Here's how the part is built. I have some questions about the finished solid (model axes, mm). A direction names the side the tool comes from. Round coordinates to 2 decimals unless told otherwise and drop trailing zeros. Write each loop counter-clockwise with the first axis right and the second up, starting at its lowest first coordinate (ties: lowest second). Pieces come first, ordered by that corner, then holes. Notation, with made-up numbers: (8.5, 22.5) - (51.5, 22.5) arc R27 ccw to (51.5, 39.5) - close; hole circle Ø10 at (6, 65.25). An arc over 180 degrees is marked (long way). One line per item, written item: value. Start each with the question number.
Item 1: If I drill on line 1 (X direction, y = 0, z = -0.2); line 2 (X direction, y = 0, z = -2.8); line 3 (Z direction, x = 2.75, y = 2.25), over which ranges is the centre line in solid material (lowest first)?
Item 2: Imagine slicing it at D-D, the plane x = -2.75. Please give me the cut outline in (y, z), then the cut area to 3 significant figures.
Item 3: For faces 3 (the face through (-2.75, 1.43, -4.05)), 4 (the face through (2.44, -0.54, -2.07)), which set-ups out of +Z, -Z, +X, -X, +Y, -Y let a thin tool reach every point of the face, with its end or its side?
Item 4: Imagine slicing it at C-C, the plane z = -1.3. Please give me the cut outline in (x, y).
Item 5: Imagine slicing it at A-A, the plane x = 0. Please give me the cut outline in (y, z).
Item 6: Thinking about a two-plate mould opening in Y: for faces 1 (the face through (-4.88, -1.08, -2.13)), 2 (the face through (2.8, -3.65, -4.05)), which applies, released by +Y, released by -Y, zero draft, split by the parting line, or undercut?
Autodesk Inventor part; units mm, degrees
ref_plane "YZ Plane" through (0, 0, 0) normal (1, 0, 0) x (0, 1, 0)
ref_plane "XZ Plane" through (0, 0, 0) normal (0, 1, 0) x (-1, 0, 0)
ref_plane "XY Plane" through (0, 0, 0) normal (0, 0, 1) x (1, 0, 0)
sketch "Sketch1" plane through (0, 0, 0) normal (1, 0, 0) x (0, 1, 0)
  line L0 (4, 0) -> (2.5, 0)
  line L1 (2.5, 0) -> (3.1, 0)
  line L2 (3.1, 0) -> (3.1, -0.3)
  line L3 (3.1, -0.3) -> (4.6, -0.3)
  line L4 (4.6, -0.3) -> (4.6, 0)
  line L5 (4.6, 0) -> (5, 0)
  line L6 (5, 0) -> (5, -4.2)
  line L7 (5, -4.2) -> (4.6, -4.2)
  line L8 (4.6, -4.2) -> (4.6, -3.9)
  line L9 (4.6, -3.9) -> (3.1, -3.9)
  line L10 (3.1, -3.9) -> (3.1, -4.2)
  line L11 (3.1, -4.2) -> (2.5, -4.2)
  line L12 (2.5, -4.2) -> (2.5, 0)
  line L13 (0, 0) -> (0, -4.97)
revolve "Revolution1" add sketch "Sketch1" angle 360 about axis through (0, 0, 0) along (0, 0, -1)
properties part number "Ball Bearing 5 x 10 x 4.2" material "Stainless Steel"
Values follow:
1. line 1: x = -5 to -4.6, -3.1 to -2.5, 2.5 to 3.1, 4.6 to 5
1. line 2: x = -5 to -2.5, 2.5 to 5
1. line 3: z = -3.9 to -0.3
2. outline: (-4.18, -4.2) - (-3.69, -4.2) - (-3.69, -3.9) - (-1.43, -3.9) - (-1.43, -4.2) - (1.43, -4.2) - (1.43, -3.9) - (3.69, -3.9) - (3.69, -4.2) - (4.18, -4.2) - (4.18, 0) - (3.69, 0) - (3.69, -0.3) - (1.43, -0.3) - (1.43, 0) - (-1.43, 0) - (-1.43, -0.3) - (-3.69, -0.3) - (-3.69, 0) - (-4.18, 0) - close
2. area: 32.4 mm^2
3. face 3: -Z
3. face 4: +Z, -Z
4. outline: circle Ø10 at (0, 0); hole circle Ø5 at (0, 0)
5. outline: (-5, -4.2) - (-4.6, -4.2) - (-4.6, -3.9) - (-3.1, -3.9) - (-3.1, -4.2) - (-2.5, -4.2) - (-2.5, 0) - (-3.1, 0) - (-3.1, -0.3) - (-4.6, -0.3) - (-4.6, 0) - (-5, 0) - close; (2.5, -4.2) - (3.1, -4.2) - (3.1, -3.9) - (4.6, -3.9) - (4.6, -4.2) - (5, -4.2) - (5, 0) - (4.6, 0) - (4.6, -0.3) - (3.1, -0.3) - (3.1, 0) - (2.5, 0) - close
6. face 1: split by the parting line
6. face 2: undercut
